Could you check a few things on this model? Use its own coordinates, in mm. A direction names the side the tool comes from. Coordinates: 2 decimals unless noted, no trailing zeros. Loops run counter-clockwise (first coordinate to the right, second up) from the corner with the lowest first, then second, coordinate; pieces in that order, holes last. Notation, with made-up numbers: (60.25, -17.5) - (77.25, -17.5) arc R15 cw to (77.25, 6.5) - close; hole circle Ø2 at (-22, -13.5). An arc over 180 degrees is marked (long way). Use CSV: the item, a comma, the result in double quotes.
from build123d import *

# Parameters (mm, degrees)
BOSS_EXTRUDE1_DEPTH = 12.7
CAVITY1_START       = 98.335975301
CAVITY1_OUTLINE_R   = 12.7
CAVITY1_DEPTH       = 41.588388123
CAVITY1_2_OUTLINE_R = 12.7
CAVITY1_2_DEPTH     = 41.588388123


# Read off the part's stored shape, not the designer's step: Cavity1
with BuildPart() as part:
    # Sketch2 → Boss-Extrude1 (new body)
    with BuildSketch(Plane(origin=(0, 230.1, 0), x_dir=(1, 0, 0), z_dir=(0, 1, 0))):
        Polygon((2540, 190.5), (2667, 190.5), (2667, 143.842086105), (2603.5, 143.842086105), (2603.5, 131.142086105), (2667, 131.142086105), (2667, -131.142086105), (2603.5, -131.142086105), (2603.5, -143.842086105), (2667, -143.842086105), (2667, -190.5), (2540, -190.5), align=None)
    extrude(amount=-BOSS_EXTRUDE1_DEPTH)

    # Cavity1 outline → Cavity1 (cut)
    with BuildSketch(Plane(origin=(0, 0, 0), x_dir=(1, 0, 0), z_dir=(0, 0.7256238511734343, -0.6880915830092923)).offset(CAVITY1_START)):
        with Locations((2600, -199.546559073)):
            Circle(CAVITY1_OUTLINE_R)
    extrude(amount=CAVITY1_DEPTH, mode=Mode.SUBTRACT)

    # Cavity1 2 outline → Cavity1 2 (cut)
    with BuildSketch(Plane(origin=(0, 0, 0), x_dir=(1, 0, 0), z_dir=(0, 0.7256238511734294, 0.6880915830092974)).offset(CAVITY1_START)):
        with Locations((2600, 199.546559073)):
            Circle(CAVITY1_2_OUTLINE_R)
    extrude(amount=CAVITY1_2_DEPTH, mode=Mode.SUBTRACT)


solid = part.part
(1) Thinking about a two-plate mould opening in Z: for faces 1 (the face through (2587.312, 223.155, 62.618)), 2 (the face through (2603, 224, -190.5)), 3 (the face through (2667, 224, -167)), 4 (the face through (2603.5, 224, -138)), which applies, +Z half, -Z half, draft (parallel to the pull), parting line (faces both ways), or undercut?
Computed:
face 1,"undercut"
face 2,"-Z half"
face 3,"draft"
face 4,"undercut"
(2) Which directions (+Z, -Z, +X, -X, +Y, -Y) give clear straight access to the entire face, cutting with the end or side of a thin tool? Please do faces 5 (the face through (2667, 224, -2)), 6 (the face through (2635, 224, 143.842)).
Computed:
face 5,"+Z, -Z, +X, +Y, -Y"
face 6,"+X, +Y, -Y"
(3) Please list where these lines run through material, in increasing order: line 1 (Z direction, x = 2635, y = 222.75); line 2 (X direction, y = 218.5, z = -76); line 3 (X direction, y = 222.75, z = -137).
Computed:
line 1,"z = -190.5 to -143.84, -131.14 to 131.14, 143.84 to 190.5"
line 2,"x = 2540 to 2588.78, 2611.22 to 2667"
line 3,"x = 2540 to 2603.5"
(4) Suppose I cut it at B-B (y = 228). State how many separate pieces and enclosed holes the cut face has, plus the area to 3 significant figures.
Computed:
separate pieces,"1"
enclosed holes,"2"
area,"45,400 mm²"
(5) Suppose I cut it at A-A (x = 2647). Write out the boundary of the cut face in (y, z).
Computed:
outline,"(217.4, -190.5) - (230.1, -190.5) - (230.1, -143.84) - (217.4, -143.84) - close; (217.4, -131.14) - (230.1, -131.14) - (230.1, 131.14) - (217.4, 131.14) - close; (217.4, 143.84) - (230.1, 143.84) - (230.1, 190.5) - (217.4, 190.5) - close"
